For this review, take the finished solid that the model builds, in its own axes (mm). Face numbers are marked on the shaded views. A direction names the side the tool comes from. Coordinates: 2 decimals unless noted, no trailing zeros. Loops run counter-clockwise (first coordinate to the right, second up) from the corner with the lowest first, then second, coordinate; pieces in that order, holes last.
```python
from build123d import *

# Parameters (mm, degrees)
IZIM1_R                                    = 22.5
IZIM1_R_2                                  = 16.25
Y_KSEKLIK_EKSTR_ZYON1_DEPTH                = 8.25
IZIM1_R_3                                  = 33.05
IZIM1_R_4                                  = 28
Y_KSEKLIK_EKSTR_ZYON1_2_DEPTH              = 8.25
IZIM2_R                                    = 2
IZIM2_R_2                                  = 1.5
IZIM2_R_3                                  = 8.25
Y_KSEKLIK_EKSTR_ZYON2_DEPTH                = 5
M4_ALT_GEN_ALYAN_HAV_A_BA_L_VIDA_I_2_COUNT = 2
M4_ALT_GEN_ALYAN_HAV_A_BA_L_VIDA_I_2_PITCH = 49.5
M4_ALT_GEN_ALYAN_HAV_A_BA_L_VIDA_I_3_COUNT = 2
M4_ALT_GEN_ALYAN_HAV_A_BA_L_VIDA_I_3_PITCH = 70.003571337
M4_ALT_GEN_ALYAN_HAV_A_BA_L_VIDA_I_4_COUNT = 2
M4_ALT_GEN_ALYAN_HAV_A_BA_L_VIDA_I_4_PITCH = 49.5
IZIM7_R                                    = 16.25
KES_EKSTR_ZYON2_DEPTH                      = 1
IZIM8_R                                    = 4.567222976
KES_EKSTR_ZYON3_DEPTH                      = 8.25


with BuildPart() as part:
    # izim1 → Y_kseklik-Ekstr_zyon1 (new body)
    with BuildSketch(Plane.XY):
        Circle(IZIM1_R)
        Circle(IZIM1_R_2, mode=Mode.SUBTRACT)
    extrude(amount=Y_KSEKLIK_EKSTR_ZYON1_DEPTH)



with BuildPart() as body_2:
    # izim1 → Y_kseklik-Ekstr_zyon1 2 (new body)
    with BuildSketch(Plane.XY):
        Circle(IZIM1_R_3)
        Circle(IZIM1_R_4, mode=Mode.SUBTRACT)
    extrude(amount=Y_KSEKLIK_EKSTR_ZYON1_2_DEPTH)


with BuildPart() as part_1:
    add(part.part)

    add(body_2.part)  # Y_kseklik-Ekstr_zyon2 merges body 2
    # izim2 → Y_kseklik-Ekstr_zyon2 (add)
    with BuildSketch(Plane.XY.offset(8.25)):
        with BuildLine():
            ThreePointArc((-10.540830255, 39.621848739), (-28.991378029, 28.991378029), (-39.621848739, 10.540830255))
            ThreePointArc((-39.621848739, 10.540830255), (-41.396931543, 6.966269622), (-44.428571429, 4.370588155))
            ThreePointArc((-44.428571429, 4.370588155), (-47, 0), (-44.428571429, -4.370588155))
            ThreePointArc((-44.428571429, -4.370588155), (-41.396931543, -6.966269622), (-39.621848739, -10.540830255))
            ThreePointArc((-39.621848739, -10.540830255), (-28.991378029, -28.991378029), (-10.540830255, -39.621848739))
            ThreePointArc((-10.540830255, -39.621848739), (-6.966269622, -41.396931543), (-4.370588155, -44.428571429))
            ThreePointArc((-4.370588155, -44.428571429), (0, -47), (4.370588155, -44.428571429))
            ThreePointArc((4.370588155, -44.428571429), (6.966269622, -41.396931543), (10.540830255, -39.621848739))
            ThreePointArc((10.540830255, -39.621848739), (28.991378029, -28.991378029), (39.621848739, -10.540830255))
            ThreePointArc((39.621848739, -10.540830255), (41.396931543, -6.966269622), (44.428571429, -4.370588155))
            ThreePointArc((44.428571429, -4.370588155), (47, 0), (44.428571429, 4.370588155))
            ThreePointArc((44.428571429, 4.370588155), (41.396931543, 6.966269622), (39.621848739, 10.540830255))
            ThreePointArc((39.621848739, 10.540830255), (28.991378029, 28.991378029), (10.540830255, 39.621848739))
            ThreePointArc((10.540830255, 39.621848739), (6.966269622, 41.396931543), (4.370588155, 44.428571429))
            ThreePointArc((4.370588155, 44.428571429), (0, 47), (-4.370588155, 44.428571429))
            ThreePointArc((-4.370588155, 44.428571429), (-6.966269622, 41.396931543), (-10.540830255, 39.621848739))
        make_face()
        with Locations(Location((-24.75, 24.75, 0), (0, 0, 302.756106046))):
            Circle(IZIM2_R, mode=Mode.SUBTRACT)
        with Locations(Location((24.75, 24.75, 0), (0, 0, 212.756106046))):
            Circle(IZIM2_R, mode=Mode.SUBTRACT)
        with Locations(Location((24.75, -24.75, 0), (0, 0, 147.243893954))):
            Circle(IZIM2_R, mode=Mode.SUBTRACT)
        with Locations(Location((-24.75, -24.75, 0), (0, 0, 57.243893954))):
            Circle(IZIM2_R, mode=Mode.SUBTRACT)
        with Locations((0, 42)):
            Circle(IZIM2_R_2, mode=Mode.SUBTRACT)
        with Locations((42, 0)):
            Circle(IZIM2_R_2, mode=Mode.SUBTRACT)
        with Locations((0, -42)):
            Circle(IZIM2_R_2, mode=Mode.SUBTRACT)
        with Locations((-42, 0)):
            Circle(IZIM2_R_2, mode=Mode.SUBTRACT)
        Circle(IZIM2_R_3, mode=Mode.SUBTRACT)
    extrude(amount=Y_KSEKLIK_EKSTR_ZYON2_DEPTH)

    # izim5 → M4 Alt_gen Alyan Hav_a Ba_l_ Vida _in Ha (revolve, cut)
    with BuildSketch(Plane(origin=(24.75, 24.75, 8.25), x_dir=(0, 1, 0), z_dir=(1, 0, 0))):
        Polygon((0, 0), (0, 5), (2.25, 5), (2.25, 2.34), (4.59, 0), align=None)
    m4_alt_gen_alyan_hav_a_ba_l_vida_in_ha = revolve(axis=Axis((24.75, 24.75, 1.9), (0, 0, 1)), mode=Mode.SUBTRACT)

    # M4 Alt_gen Alyan Hav_a Ba_l_ Vida _i 2: M4 Alt_gen Alyan Hav_a Ba_l_ Vida _in Ha ×2
    with Locations(*[(-i * M4_ALT_GEN_ALYAN_HAV_A_BA_L_VIDA_I_2_PITCH, 0, 0) for i in range(1, M4_ALT_GEN_ALYAN_HAV_A_BA_L_VIDA_I_2_COUNT)]):
        add(m4_alt_gen_alyan_hav_a_ba_l_vida_in_ha, mode=Mode.SUBTRACT)

    # M4 Alt_gen Alyan Hav_a Ba_l_ Vida _i 3: M4 Alt_gen Alyan Hav_a Ba_l_ Vida _in Ha ×2
    with Locations(*[Vector(-0.7071067811865475, -0.7071067811865476, 0) * (i * M4_ALT_GEN_ALYAN_HAV_A_BA_L_VIDA_I_3_PITCH) for i in range(1, M4_ALT_GEN_ALYAN_HAV_A_BA_L_VIDA_I_3_COUNT)]):
        add(m4_alt_gen_alyan_hav_a_ba_l_vida_in_ha, mode=Mode.SUBTRACT)

    # M4 Alt_gen Alyan Hav_a Ba_l_ Vida _i 4: M4 Alt_gen Alyan Hav_a Ba_l_ Vida _in Ha ×2
    with Locations(*[(0, -i * M4_ALT_GEN_ALYAN_HAV_A_BA_L_VIDA_I_4_PITCH, 0) for i in range(1, M4_ALT_GEN_ALYAN_HAV_A_BA_L_VIDA_I_4_COUNT)]):
        add(m4_alt_gen_alyan_hav_a_ba_l_vida_in_ha, mode=Mode.SUBTRACT)

    # izim7 → Kes-Ekstr_zyon2 (cut)
    with BuildSketch(Plane(origin=(0, 0, 8.25), x_dir=(-1, 0, 0), z_dir=(0, 0, -1))):
        Circle(IZIM7_R)
    extrude(amount=-KES_EKSTR_ZYON2_DEPTH, mode=Mode.SUBTRACT)

    # izim8 → Kes-Ekstr_zyon3 (cut)
    with BuildSketch(Plane(origin=(0, 0, 0), x_dir=(-1, 0, 0), z_dir=(0, 0, -1))):
        with Locations((-24.75, 24.75)):
            Circle(IZIM8_R)
        with Locations((24.75, 24.75)):
            Circle(IZIM8_R)
        with Locations((24.75, -24.75)):
            Circle(IZIM8_R)
        with Locations((-24.75, -24.75)):
            Circle(IZIM8_R)
    extrude(amount=-KES_EKSTR_ZYON3_DEPTH, mode=Mode.SUBTRACT)


solid = part_1.part
```
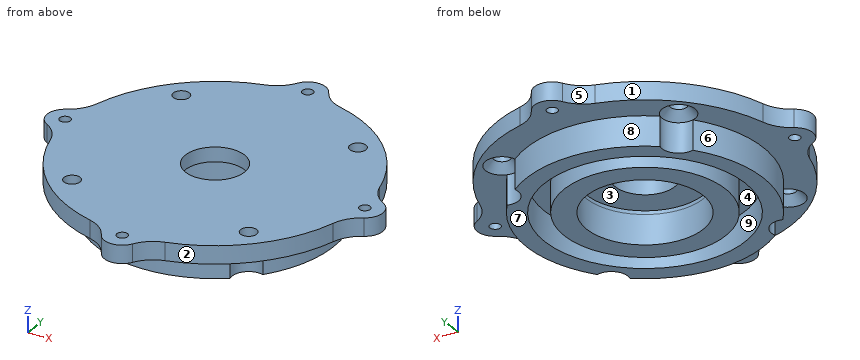
Q1. The part is to be moulded in two halves that separate along X. For the marked faces 1, 2, 3 and 4, say which applies: +X half, -X half, draft (parallel to the pull), parting line (faces both ways), or undercut.
Q2. For pin 1 Ø4 at (y, z) = (21.5, 6) entering from -X; pin 2 Ø2 at (x, y) = (22.5, 7.5) entering from -Z; pin 3 Ø4 at (y, z) = (18, 10) entering from +X, all flat-tipped, find the tip position at first contact; note any pin that passes through.
Q3. Wall thickness on probe 1 along Y at (x, z) = (0, 8.5); probe 2 along Y at (x, z) = (0, 1.5); probe 3 along X at (y, z) = (24.75, 11.95): over which ranges is each line inside the solid? List them lowest first.
Q4. Consider section B-B (x = 0). Count the separate pieces of the cut face and the enclosed holes in it, then the cut area to 3 significant figures.
Q5. Machinability: for the marked faces 5, 6, 7, 8 and 9, which of the approach directions +Z, -Z, +X, -X, +Y, -Y give a long, thin tool a straight path to every point of the face, cutting with its end or side? Answer none if there is none.
Q6. Consider section C-C (y = 42). State the section outline as (x, z) points, then the cut area to 3 significant figures.
Q7. Consider section A-A (z = 5). State the section outline as (x, y) points, then the cut area to 3 significant figures.
Model answer:
1. face 1: -X half
1. face 2: +X half
1. face 3: undercut
1. face 4: undercut
2. pin 1: stops at x = -26.68
2. pin 2: stops at z = 8.25
2. pin 3: stops at x = 37.75
3. probe 1: y = -47 to -43.5, -40.5 to -16.25, 16.25 to 40.5, 43.5 to 47
3. probe 2: y = -33.05 to -28, -22.5 to -16.25, 16.25 to 22.5, 28 to 33.05
3. probe 3: x = -32.69 to -27, -22.5 to 22.5, 27 to 32.69
4. separate pieces: 4
4. enclosed holes: 0
4. area: 528 mm2
5. face 5: +Z, -Z, -X, +Y
5. face 6: -Z, -X
5. face 7: -Z, +X, -X, +Y, -Y
5. face 8: -Z, +Y
5. face 9: -Z
6. outline: (-6.26, 8.25) - (-1.5, 8.25) - (-1.5, 13.25) - (-6.26, 13.25) - close; (1.5, 8.25) - (6.26, 8.25) - (6.26, 13.25) - (1.5, 13.25) - close
6. area: 47.6 mm2
7. outline: (-26.03, -20.37) arc R4.57 cw to (-20.37, -26.03) arc R33.05 ccw to (20.37, -26.03) arc R4.57 cw to (26.03, -20.37) arc R33.05 ccw to (26.03, 20.37) arc R4.57 cw to (20.37, 26.03) arc R33.05 ccw to (-20.37, 26.03) arc R4.57 cw to (-26.03, 20.37) arc R33.05 ccw to start; circle Ø45 at (0, 0); hole circle Ø56 at (0, 0); hole circle Ø32.5 at (0, 0)
7. area: 1,670 mm2
